Build history of the part. All positions in model axes, mm. Give positions to 0.01 mm unless a question says otherwise; leave off trailing zeros. Order: outer loops, then holes, each group sorted by start corner. A loop starts at its lowest first (then second) coordinate and runs counter-clockwise, first axis right, second up. Notation, with made-up numbers: (33.5, -2.5) - (42.5, -2.5) arc R22 cw to (42.5, 3.5) - close; hole circle Ø6 at (2, 21). An arc over 180 degrees is marked (long way). Write each question's results on one line, items separated by ' | '. Start each with the question number.
1) Cut at A-A on z = -11. List the corners of the cut face in (x, y), plus the area to 3 significant figures.
2) Two-plate mould, pull along Y, no slides. Class faces 1 (the face through (0, 0, 0)), 2 (the face through (17.53, 5.4, -0.32)), 3 (the face through (14.88, 2.39, 0.32)), 4 (the face through (18.1, 2, 0)): +Y half, -Y half, draft (parallel to the pull), parting line (faces both ways), or undercut.
3) Drill centre lines: line 1 along Y through (x, z) = (13.4, 12); line 2 along X through (y, z) = (1.8, 19); line 3 along Y through (x, z) = (-13, -6). Where is each one in solid material? Low to high. Write a range as from..to.
4) Cut at D-D on y = 5.35. List the corners of the cut face in (x, z).
5) Cut at C-C on x = 13.4. List the corners of the cut face in (y, z).
6) Drop a flat-ended pin along its axis: pin 1 Ø1 at (x, z) = (-7.5, -16) entering from -Y. Give the stop position or say it passes through.
7) Cut at B-B on y = 3. List the corners of the cut face in (x, z).
from build123d import *

# Parameters (mm, degrees)
SKETCH1_W           = 36.2
SKETCH1_H           = 45
BOSS_EXTRUDE1_DEPTH = 6
FILLET1_R           = 2
SKETCH3_R           = 1.6
CUT_EXTRUDE1_DEPTH  = 49.873407902


with BuildPart() as part:
    # Sketch1 → Boss-Extrude1 (new body)
    with BuildSketch(Plane(origin=(0, 0, 0), x_dir=(1, 0, 0), z_dir=(0, 1, 0))):
        Rectangle(SKETCH1_W, SKETCH1_H)
    extrude(amount=BOSS_EXTRUDE1_DEPTH)

    # Fillet1
    fillet1_edges = [part.edges().sort_by_distance(p)[0] for p in [
        (-18.1, 6, 0),
        (18.1, 6, 0),
    ]]
    fillet(fillet1_edges, radius=FILLET1_R)

    # Sketch3 → Cut-Extrude1 (cut, through all)
    with BuildSketch(Plane.XY.offset(22.5)):
        with Locations((-13.4, 3)):
            Circle(SKETCH3_R)
        with Locations((13.4, 3)):
            Circle(SKETCH3_R)
    extrude(amount=-CUT_EXTRUDE1_DEPTH, mode=Mode.SUBTRACT)


solid = part.part
Results:
1) outline: (-18.1, 0) - (18.1, 0) - (18.1, 4) arc R2 ccw to (16.1, 6) - (-16.1, 6) arc R2 ccw to (-18.1, 4) - close; hole circle Ø3.2 at (-13.4, 3); hole circle Ø3.2 at (13.4, 3) | area: 199 mm^2
2) face 1: -Y half | face 2: +Y half | face 3: undercut | face 4: draft
3) line 1: 0..1.4, 4.6..6 | line 2: -18.1..-14.46, -12.34..12.34, 14.46..18.1 | line 3: 0..1.45, 4.55..6
4) outline: (-17.58, -22.5) - (17.58, -22.5) - (17.58, 22.5) - (-17.58, 22.5) - close
5) outline: (0, -22.5) - (1.4, -22.5) - (1.4, 22.5) - (0, 22.5) - close; (4.6, -22.5) - (6, -22.5) - (6, 22.5) - (4.6, 22.5) - close
6) pin 1: y = 0
7) outline: (-18.1, -22.5) - (-15, -22.5) - (-15, 22.5) - (-18.1, 22.5) - close; (-11.8, -22.5) - (11.8, -22.5) - (11.8, 22.5) - (-11.8, 22.5) - close; (15, -22.5) - (18.1, -22.5) - (18.1, 22.5) - (15, 22.5) - close
